```python
from build123d import *

# Parameters (mm, degrees)
SKETCH2_W          = 47.16496854
SKETCH2_H          = 39.085316542
CUT_EXTRUDE1_DEPTH = 5.61
SKETCH3_W          = 40
SKETCH3_H          = 40
CUT_EXTRUDE2_DEPTH = 50


with BuildPart() as part:
    # Sketch1 → Revolve1 (revolve)
    with BuildSketch(Plane.XY):
        Polygon((0, 34.0386), (5.5795, 34.0386), (5.5795, 14.2396), (5.682246885, 11.4036), (12.7, 11.4036), (17.933402515, 8.382093649), (13.45, 5.7936), (0, 5.7936), align=None)
    revolve(axis=Axis((0, 5.7936, 0), (0, 1, 0)))

    # Sketch2 → Cut-Extrude1 (cut)
    with BuildSketch(Plane(origin=(0, 11.4036, 0), x_dir=(1, 0, 0), z_dir=(0, 1, 0))):
        with Locations((0.151493475, -0.8079652)):
            Rectangle(SKETCH2_W, SKETCH2_H)
        Polygon((14.664696837, 0), (7.332348419, 12.7), (-7.332348419, 12.7), (-14.664696837, 0), (-7.332348419, -12.7), (7.332348419, -12.7), align=None, mode=Mode.SUBTRACT)
    extrude(amount=-CUT_EXTRUDE1_DEPTH, mode=Mode.SUBTRACT)

    # Sketch3 → Cut-Extrude2 (cut)
    with BuildSketch(Plane(origin=(0, 14.0616, 0), x_dir=(1, 0, 0), z_dir=(0, 1, 0))):
        Rectangle(SKETCH3_W, SKETCH3_H)
    extrude(amount=CUT_EXTRUDE2_DEPTH, mode=Mode.SUBTRACT)


solid = part.part
```
The model under review builds one solid part; all positions refer to its coordinate system, in mm. A direction names the side the tool comes from. Coordinates: 2 decimals unless noted, no trailing zeros. Write each loop counter-clockwise with the first axis right and the second up, starting at its lowest first coordinate (ties: lowest second). Pieces come first, ordered by that corner, then holes.
1) We need section B-B on y = 12. State the section outline as (x, z) points, then the cut area to 3 significant figures.
2) We need section A-A on y = 7.5. State the section outline as (x, z) points, then the cut area to 3 significant figures.
3) Machinability: for faces 1 (the face through (-5.5, 11.404, 2.6)), 2 (the face through (-6.561, 11.128, -11.428)), which of the approach directions +Z, -Z, +X, -X, +Y, -Y give a long, thin tool a straight path to every point of the face, cutting with its end or side? Answer none if there is none.
4) To check wall thickness, follow probe 1 along Y at (x, z) = (-2.25, -6.75); probe 2 along X at (y, z) = (12.5, 3.5); probe 3 along Z at (x, y) = (-13.5, 8.25). State the ranges of each line that lie inside material, in increasing order.
5) Clearance check with flat-ended pins moving along their axes: pin 1 Ø1 at (x, z) = (-6.5, -3.5) entering from +Y; pin 2 Ø4 at (y, z) = (8.5, 1) entering from -X. State where each tip first meets the part, or that it passes through.
Answer list:
1. outline: circle Ø11.32 at (0, 0)
1. area: 101 mm2
2. outline: (-14.66, 0) - (-7.33, -12.7) - (7.33, -12.7) - (14.66, 0) - (7.33, 12.7) - (-7.33, 12.7) - close
2. area: 559 mm2
3. face 1: +Y
3. face 2: -Z, -X, +Y
4. probe 1: y = 5.79 to 11.4
4. probe 2: x = -4.43 to 4.43
4. probe 3: z = -2.02 to 2.02
5. pin 1: stops at y = 11.4
5. pin 2: stops at x = -14.66
